Check sheet for the modelled part. Datum: model origin and axes. Units: mm. A direction names the side the tool comes from. Round coordinates to 2 decimals unless told otherwise and drop trailing zeros. Write each loop counter-clockwise with the first axis right and the second up, starting at its lowest first coordinate (ties: lowest second). Pieces come first, ordered by that corner, then holes.
Item 1: Cross-section at C-C on x = -3.5. Enter the section's corners in (y, z), plus the area to 3 significant figures.
Item 2: Material ranges on line 1 (X direction, y = 3.65, z = 0); line 2 (Y direction, x = 1, z = 0), recorded low to high.
Item 3: Cross-section at A-A on x = -0.75. Enter the section's corners in (y, z).
Item 4: Tool access check on faces 1 (the flat face through (-3, 2, -3)), 2 (the flat face through (3, 2, 3)), 3 (the cylindrical face through (-3, 3, 0)). Record the directions out of +Z, -Z, +X, -X, +Y, -Y that give a thin tool (end or side, any length) a straight path to the whole face; none if there is none.
Item 5: Cross-section at B-B on z = 2. Enter the section's corners in (x, y), plus the area to 3 significant figures.
from build123d import *

# Parameters (mm, degrees)
IZIM1_W                     = 8
IZIM1_H                     = 8
Y_KSEKLIK_EKSTR_ZYON1_DEPTH = 2
IZIM2_R                     = 4
IZIM2_R_2                   = 3
EKSTR_ZYON_NCE1_DEPTH       = 3


with BuildPart() as part:
    # Çizim1 → Yükseklik-Ekstrüzyon1 (new body)
    with BuildSketch(Plane(origin=(0, 0, 0), x_dir=(1, 0, 0), z_dir=(0, 1, 0))):
        Rectangle(IZIM1_W, IZIM1_H)
    extrude(amount=Y_KSEKLIK_EKSTR_ZYON1_DEPTH)

    # Çizim2 → Ekstrüzyon-İnce1 (add)
    with BuildSketch(Plane(origin=(0, 2, 0), x_dir=(1, 0, 0), z_dir=(0, 1, 0))):
        Circle(IZIM2_R)
        Circle(IZIM2_R_2, mode=Mode.SUBTRACT)
    extrude(amount=EKSTR_ZYON_NCE1_DEPTH)


solid = part.part
Response values:
1. outline: (0, -4) - (2, -4) - (2, -1.94) - (5, -1.94) - (5, 1.94) - (2, 1.94) - (2, 4) - (0, 4) - close
1. area: 27.6 mm2
2. line 1: x = -4 to -3, 3 to 4
2. line 2: y = 0 to 2
3. outline: (0, -4) - (2, -4) - (2, -3.93) - (5, -3.93) - (5, -2.9) - (2, -2.9) - (2, 2.9) - (5, 2.9) - (5, 3.93) - (2, 3.93) - (2, 4) - (0, 4) - close
4. face 1: -Z, -X, +Y
4. face 2: +Z, +X, +Y
4. face 3: +Y
5. outline: (-4, 0) - (4, 0) - (4, 2) - (3.46, 2) - (3.46, 5) - (2.24, 5) - (2.24, 2) - (-2.24, 2) - (-2.24, 5) - (-3.46, 5) - (-3.46, 2) - (-4, 2) - close
5. area: 23.4 mm2
